```python
from build123d import *

# Parameters (mm, degrees)
BOSS_EXTRUDE1_DEPTH = 250
SKETCH3_W           = 5
SKETCH3_H           = 100
CUT_EXTRUDE1_DEPTH  = 250
SKETCH4_W           = 5
SKETCH4_H           = 250
BOSS_EXTRUDE2_DEPTH = 160


with BuildPart() as part:
    # Sketch1 → Boss-Extrude1 (new body)
    with BuildSketch(Plane(origin=(0, 0, 0), x_dir=(1, 0, 0), z_dir=(0, 1, 0))):
        Polygon((-250, 0), (-250, 500), (250, 500), (250, 0), (245, 0), (245, 495), (-245, 495), (-245, 0), align=None)
    extrude(amount=BOSS_EXTRUDE1_DEPTH)

    # Sketch3 → Cut-Extrude1 (cut)
    with BuildSketch(Plane(origin=(0, 250, 0), x_dir=(1, 0, 0), z_dir=(0, 1, 0))):
        with Locations((247.5, 50)):
            Rectangle(SKETCH3_W, SKETCH3_H)
    extrude(amount=-CUT_EXTRUDE1_DEPTH, mode=Mode.SUBTRACT)

    # Sketch4 → Boss-Extrude2 (add)
    with BuildSketch(Plane.XY):
        with Locations((-247.5, 125)):
            Rectangle(SKETCH4_W, SKETCH4_H)
    extrude(amount=BOSS_EXTRUDE2_DEPTH)


solid = part.part
```
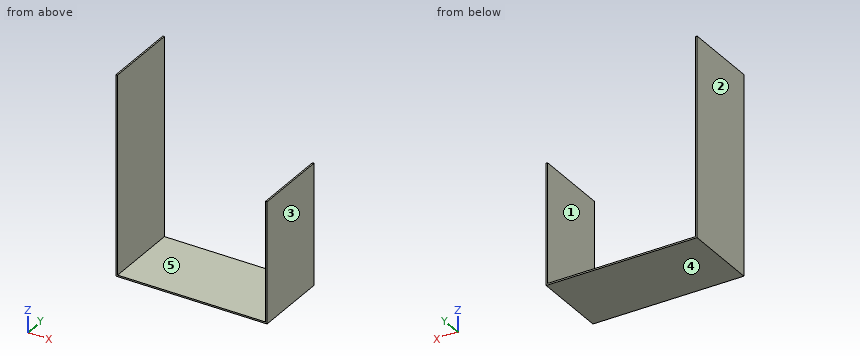
The listing builds one solid part. Answer for the finished solid, in the listing's coordinates (mm). Face numbers are marked on the shaded views. A direction names the side the tool comes from. Give positions to 0.01 mm unless a question says otherwise; leave off trailing zeros. Write each loop counter-clockwise with the first axis right and the second up, starting at its lowest first coordinate (ties: lowest second). Pieces come first, ordered by that corner, then holes. Notation, with made-up numbers: (7, 70.25) -> (14, 70.25) arc R20 cw to (14, 100.25) -> close; hole circle Ø3 at (7, -3). An arc over 180 degrees is marked (long way). Write item = value, one per line. Start each with the question number.
1) Determine the mould class of the marked faces 1, 2 and 3 for opening direction X: +X half, -X half, draft (parallel to the pull), parting line (faces both ways), or undercut.
2) Straight lines are drawn through the part: line 1 along X through (y, z) = (78, -222); line 2 along Z through (x, y) = (-186.5, 134); line 3 along X through (y, z) = (46.5, 115). For each, find the intervals that lie inside material, in ascending order.
3) The part is cut by section A-A, the plane z = -359. Determine the outline of the cut face in (x, y), and give its area (3 significant figures).
4) Which of the six approach directions +Z, -Z, +X, -X, +Y, -Y give full straight-line access (tool end or side, diameter ignored) to the marked faces 4 and 5?
5) The part is cut by section B-B, the plane y = 183.5. Determine the outline of the cut face in (x, z), and give its area (3 significant figures).
6) The part is cut by section C-C, the plane x = -169.5. Determine the outline of the cut face in (y, z), and give its area (3 significant figures).
7) The part is cut by section D-D, the plane z = 68.5. Determine the outline of the cut face in (x, y), and give its area (3 significant figures).
8) Each of these flat-tipped pins is pushed along its axis until it touches: pin 1 (4 mm diameter, centred on x = 246.5, y = 63, fed in from +Z); pin 2 (6 mm diameter, centred on x = -157.5, y = 196, fed in from +Z). Where does it stop, or does it pass through?
Solutions:
q1.face_1 = undercut
q1.face_2 = -X half
q1.face_3 = +X half
q2.line_1 = -250 to -245, 245 to 250
q2.line_2 = -500 to -495
q2.line_3 = -250 to -245
q3.outline = (-250, 0) -> (-245, 0) -> (-245, 250) -> (-250, 250) -> close; (245, 0) -> (250, 0) -> (250, 250) -> (245, 250) -> close
q3.area = 2,500 mm²
q4.face_4 = -Z, +X, -X, +Y, -Y
q4.face_5 = +Z, +Y, -Y
q5.outline = (-250, -500) -> (250, -500) -> (250, -100) -> (245, -100) -> (245, -495) -> (-245, -495) -> (-245, 160) -> (-250, 160) -> close
q5.area = 7,750 mm²
q6.outline = (0, -500) -> (250, -500) -> (250, -495) -> (0, -495) -> close
q6.area = 1,250 mm²
q7.outline = (-250, 0) -> (-245, 0) -> (-245, 250) -> (-250, 250) -> close
q7.area = 1,250 mm²
q8.pin_1 = -100
q8.pin_2 = -495
